Source: CAD feature listing. Evaluate the final solid. Frame: model axes, mm. Face numbers are marked on the shaded views. Coordinates: 2 decimals unless noted, no trailing zeros. Order: outer loops, then holes, each group sorted by start corner. A loop starts at its lowest first (then second) coordinate and runs counter-clockwise, first axis right, second up. Notation, with made-up numbers: (88.25, 51) -> (145.25, 51) arc R31 ccw to (145.25, 86) -> close; hole circle Ø10 at (-29.5, -39.75). An arc over 180 degrees is marked (long way). Put each result on its own line as item: value.
from build123d import *

# Parameters (mm, degrees)
SKETCH_1_R          = 1.5
SKETCH_1_R_2        = 11.5
EXTRUDE_1_DEPTH     = 4
CUT_EXTRUDE_1_DEPTH = 4


with BuildPart() as part:
    # 草图1 → 凸台-拉伸1 (new body)
    with BuildSketch(Plane.XY):
        Polygon((22.5, -27), (-22.5, -27), (-27.5, -27), (-27.5, -23), (-22.5, -23), (-22.5, -15), (-18.5, -15), (-18.5, -16.3), (-15.8, -16.3), (-15.8, -15), (-13.1, -15), (-13.1, -12), (-15.8, -12), (-15.8, -10.7), (-18.5, -10.7), (-18.5, -12), (-22.5, -12), (-22.5, -4), (-27.5, -4), (-27.5, 4), (-22.5, 4), (-22.5, 12), (-18.5, 12), (-18.5, 10.7), (-15.8, 10.7), (-15.8, 12), (-13.1, 12), (-13.1, 15), (-15.8, 15), (-15.8, 16.3), (-18.5, 16.3), (-18.5, 15), (-22.5, 15), (-22.5, 23), (-27.5, 23), (-27.5, 27), (-22.5, 27), (22.5, 27), (27.5, 27), (27.5, 23), (22.5, 23), (22.5, 15), (18.5, 15), (18.5, 16.3), (15.8, 16.3), (15.8, 15), (13.1, 15), (13.1, 12), (15.8, 12), (15.8, 10.7), (18.5, 10.7), (18.5, 12), (22.5, 12), (22.5, 4), (27.5, 4), (27.5, -4), (22.5, -4), (22.5, -12), (18.5, -12), (18.5, -10.7), (15.8, -10.7), (15.8, -12), (13.1, -12), (13.1, -15), (15.8, -15), (15.8, -16.3), (18.5, -16.3), (18.5, -15), (22.5, -15), (22.5, -23), (27.5, -23), (27.5, -27), align=None)
        with Locations((14, 0)):
            Circle(SKETCH_1_R, mode=Mode.SUBTRACT)
        Circle(SKETCH_1_R_2, mode=Mode.SUBTRACT)
        with Locations((0, -14)):
            Circle(SKETCH_1_R, mode=Mode.SUBTRACT)
        with Locations((-14, 0)):
            Circle(SKETCH_1_R, mode=Mode.SUBTRACT)
        with Locations((0, 14)):
            Circle(SKETCH_1_R, mode=Mode.SUBTRACT)
    extrude(amount=EXTRUDE_1_DEPTH)

    # 草图4 → 切除-拉伸1 (cut)
    with BuildSketch(Plane(origin=(0, 0, 0), x_dir=(-1, 0, 0), z_dir=(0, 0, -1))):
        Polygon((-26.5, 4), (-27.5, 3), (-27.5, 4), align=None)
        Polygon((-27.5, -3), (-26.5, -4), (-27.5, -4), align=None)
        Polygon((-27.5, -23), (-26.5, -23), (-27.5, -24), align=None)
        Polygon((-27.5, 24), (-26.5, 23), (-27.5, 23), align=None)
        Polygon((27.5, 23), (27.5, 24), (26.5, 23), align=None)
        Polygon((27.5, -24), (27.5, -23), (26.5, -23), align=None)
        Polygon((27.5, -4), (27.5, -3), (26.5, -4), align=None)
        Polygon((27.5, 4), (26.5, 4), (27.5, 3), align=None)
    extrude(amount=-CUT_EXTRUDE_1_DEPTH, mode=Mode.SUBTRACT)


solid = part.part
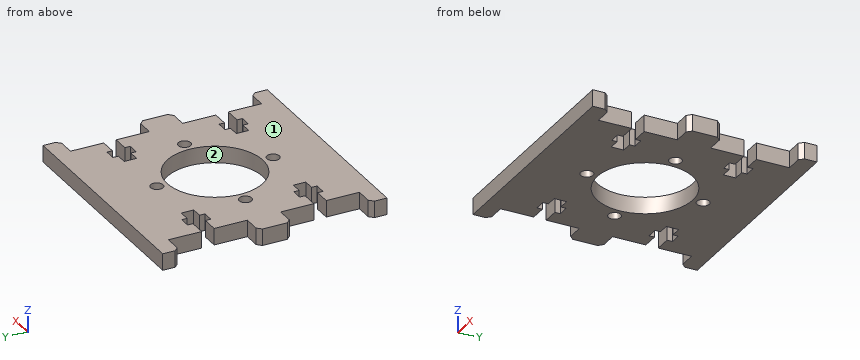
1. Ray query, line 1 along Y through (x, z) = (-14, 1.2); line 2 along Y through (x, z) = (0, 2.55); line 3 along Y through (x, z) = (20, 0.8). Return the intervals inside material, ascending.
Numbers:
line 1: y = -27 to -15, -12 to -1.5, 1.5 to 12, 15 to 27
line 2: y = -27 to -15.5, -12.5 to -11.5, 11.5 to 12.5, 15.5 to 27
line 3: y = -27 to -15, -12 to 12, 15 to 27
2. Cut plane B-B on y = -14. Output: boundary loops of the cut face in (x, z), plus the area to 3 significant figures.
Numbers:
outline: (-13.1, 0) -> (-1.5, 0) -> (-1.5, 4) -> (-13.1, 4) -> close; (1.5, 0) -> (13.1, 0) -> (13.1, 4) -> (1.5, 4) -> close
area: 92.8 mm2
3. Cut plane A-A on x = -17. Output: boundary loops of the cut face in (y, z).
Numbers:
outline: (-27, 0) -> (-16.3, 0) -> (-16.3, 4) -> (-27, 4) -> close; (-10.7, 0) -> (10.7, 0) -> (10.7, 4) -> (-10.7, 4) -> close; (16.3, 0) -> (27, 0) -> (27, 4) -> (16.3, 4) -> close
4. Pull-direction query (X, two-part tool) for the marked faces 1 and 2; classes: pulls with the +X half, pulls with the -X half, needs draft (parallel to the pull), parting line crosses it, or undercut.
Numbers:
face 1: needs draft
face 2: undercut
5. Cut plane D-D on y = 0. Output: boundary loops of the cut face in (x, z), plus the area to 3 significant figures.
Numbers:
outline: (-27.5, 0) -> (-15.5, 0) -> (-15.5, 4) -> (-27.5, 4) -> close; (-12.5, 0) -> (-11.5, 0) -> (-11.5, 4) -> (-12.5, 4) -> close; (11.5, 0) -> (12.5, 0) -> (12.5, 4) -> (11.5, 4) -> close; (15.5, 0) -> (27.5, 0) -> (27.5, 4) -> (15.5, 4) -> close
area: 104 mm2
6. First-contact query: pin 1 (1.2 mm diameter, centred on y = -8, z = 2.5, fed in from -X); pin 2 (1 mm diameter, centred on y = 15.5, z = 2, fed in from +X). Flat tips, straight axial feed; report the tip coordinate or a pass-through.
Numbers:
pin 1: stops at x = -22.5
pin 2: stops at x = 22.5
7. Cut plane C-C on x = 0. Output: boundary loops of the cut face in (y, z).
Numbers:
outline: (-27, 0) -> (-15.5, 0) -> (-15.5, 4) -> (-27, 4) -> close; (-12.5, 0) -> (-11.5, 0) -> (-11.5, 4) -> (-12.5, 4) -> close; (11.5, 0) -> (12.5, 0) -> (12.5, 4) -> (11.5, 4) -> close; (15.5, 0) -> (27, 0) -> (27, 4) -> (15.5, 4) -> close
